Autodesk Inventor part; units mm, degrees
ref_plane "Work Plane1" through (-6.76, 0, 0) normal (-1, 0, 0) x (0, -1, 0)
ref_plane "XZ Plane" through (0, 0, 0) normal (0, 1, 0) x (-1, 0, 0)
ref_plane "XY Plane" through (0, 0, 0) normal (0, 0, 1) x (1, 0, 0)
sketch "Sketch1" plane through (0, 0, 0) normal (0, 0, 1) x (1, 0, 0)
  line L0 (0, 0) -> (0, 66.5)
  line L1 (3.2, 0) -> (4, 0)
  line L2 (4, 0) -> (4, 5.9)
  line L3 (4, 5.9) -> (3.4, 6.5)
  line L4 (3.4, 6.5) -> (3.4, 45.3)
  line L5 (3.4, 45.3) -> (4, 45.9)
  line L6 (4, 45.9) -> (4, 66.5)
  line L7 (4, 66.5) -> (3.2, 66.5)
  line L8 (3.2, 66.5) -> (3.2, 0)
  dimension "d0" = 45
  dimension "d1" = 45
  dimension "d2" = 6.4
  dimension "d3" = 8
  dimension "d4" = 6.5
  dimension "d5" = 45.3
  dimension "d6" = 66.5
  dimension "d7" = 6.8
revolve "Revolution1" add sketch "Sketch1" angle 360 about axis through (0, 0, 0) along (0, 1, 0)
ref_plane "Work Plane1" through (-6.76, 0, 0) normal (-1, 0, 0) x (0, -1, 0)
sketch "Sketch2" plane through (-6.76, 0, 0) normal (-1, 0, 0) x (0, -1, 0)
  line L0 (-65.7, 1.5) -> (-54.5, 1.5)
  line L1 (-54.5, 1.5) -> (-54.5, -1.5)
  line L2 (-54.5, -1.5) -> (-65.7, -1.5)
  line L3 (-65.7, -1.5) -> (-65.7, 1.5)
  line L4 (-65.7, 2.75) -> (-54.5, 2.75)
  line L5 (-54.5, 2.75) -> (-54.5, -2.75)
  line L6 (-54.5, -2.75) -> (-65.7, -2.75)
  line L7 (-65.7, -2.75) -> (-65.7, 2.75)
  line L8 (13.7787, 0) -> (-82.6723, 0)
  line L9 (0, -4) -> (0, 4)
  dimension "d10" = 54.5
  dimension "d11" = 65.7
  dimension "d12" = 5.5
  dimension "d13" = 3
extrude "Extrusion1" add sketch "Sketch2" against normal up to surface
extrude "Extrusion2" cut sketch "Sketch2" against normal blind 1 contours L7 L4 L5 L0 | L2 L5 L6 L7
sketch "Sketch3" plane through (-5.76, 0, 0) normal (-1, 0, 0) x (0, 0, 1)
  line L0 (-1.5, 65.7) -> (-1.5, 54.5)
  line L1 (-2.75, 65.7) -> (-1.5, 65.7)
  line L2 (-2.75, 54.5) -> (-2.75, 65.7)
  line L3 (-1.5, 54.5) -> (-2.75, 54.5)
  line L4 (1.5, 54.5) -> (1.5, 65.7)
  line L5 (2.75, 54.5) -> (1.5, 54.5)
  line L6 (2.75, 65.7) -> (2.75, 54.5)
  line L7 (1.5, 65.7) -> (2.75, 65.7)
  line L8 (-4, 66.5) -> (4, 66.5)
  line L9 (2.75, 65.7) -> (-2.75, 65.7)
  line L10 (-2.75, 65.7) -> (-2.75, 66.5)
  line L11 (-2.75, 66.5) -> (2.75, 66.5)
  line L12 (2.75, 66.5) -> (2.75, 65.7)
extrude "Extrusion3" add sketch "Sketch3" against normal up to surface contours L1 L10 L8 L12 L7 L9
sketch "Sketch4" plane through (0, 66.5, 0) normal (0, 1, 0) x (1, 0, 0)
  line L0 (-5.76, 1.5) -> (-5.76, 2.75)
  line L1 (-5.76, 2.25) -> (-4.06, 2.25)
  line L2 (-4.06, 2.25) -> (-4.06, -2.25)
  line L3 (-4.06, -2.25) -> (-5.76, -2.25)
  line L4 (-5.76, -2.75) -> (-5.76, 2.75)
  line L5 (-4.76, 2.25) -> (-4.76, -2.25)
  line L6 (-8.912, 0) -> (6.152, 0)
  line L7 (-5.76, 2.25) -> (-5.76, -2.25)
  point P0 (0, 0)
  dimension "d20" = 4.06
  dimension "d21" = 4.76
  dimension "d22" = 4.5
extrude "Extrusion4" cut sketch "Sketch4" against normal up to surface (0.8 mm away) contours L0 L1 L5 L6 L4 | L6 L5 L3 L4
extrude "Extrusion5" cut sketch "Sketch4" against normal blind 9 contours L1 L2 L6 L5 | L6 L2 L3 L5
equation "\"d1\" = d0"
properties part number "PP-12" material "ABS Plastic"
Model file for the job. Use its own axes, mm. A direction names the side the tool comes from. Give positions to 0.01 mm unless a question says otherwise; leave off trailing zeros. Loops run counter-clockwise (first coordinate to the right, second up) from the corner with the lowest first, then second, coordinate; pieces in that order, holes last.
1) Flat gauge pins, fed straight in: pin 1 Ø1 at (x, z) = (-6, 0.5) entering from +Y; pin 2 Ø2 at (x, y) = (-3.5, 7.5) entering from +Z; pin 3 Ø2 at (x, y) = (-2.5, 27) entering from +Z. Where does each tip first touch, or does it go through?
2) Saw through at D-D (y = 52.5). Write the cut outline in (x, z).
3) Saw through at C-C (y = 22). Write the cut outline in (x, z).
4) Saw through at B-B (z = 0). Write the cut outline in (x, y).
5) Pull direction Z, two halves, no side cores. Call faces 4 (the flat face through (-4, 61, 2.75)), 5 (the flat face through (-5.76, 61, -2)), 6 (the flat face through (-4.5, 62.1, 2.25)): +Z half, -Z half, draft (parallel to the pull), parting line (faces both ways), or undercut.
6) Tool access for faces 1 (the flat face through (-4.5, 62.1, -2.25)), 2 (the cylindrical face through (-0.74, 26.17, 3.32)), 3 (the cylindrical face through (3.695, 56.344, 1.532)): list every direction of +Z, -Z, +X, -X, +Y, -Y with a clear straight run to the whole face (end or side of a thin tool).
7) Wall check: line 1 (Z direction, x = 0, y = 39); line 2 (Z direction, x = 0, y = 52). Give the ranges that are in metal, low to high.
8) Saw through at A-A (x = 0). Write the cut outline in (y, z).
Answer block:
1. pin 1: stops at y = 65.7
1. pin 2: stops at z = 2.3
1. pin 3: stops at z = 3.05
2. outline: circle Ø8 at (0, 0); hole circle Ø6.4 at (0, 0)
3. outline: circle Ø6.8 at (0, 0); hole circle Ø6.4 at (0, 0)
4. outline: (-6.76, 54.5) - (-4, 54.5) - (-4, 45.9) - (-3.4, 45.3) - (-3.4, 6.5) - (-4, 5.9) - (-4, 0) - (-3.2, 0) - (-3.2, 66.5) - (-4.06, 66.5) - (-4.06, 57.5) - (-4.76, 57.5) - (-4.76, 65.7) - (-6.76, 65.7) - close; (3.2, 0) - (4, 0) - (4, 5.9) - (3.4, 6.5) - (3.4, 45.3) - (4, 45.9) - (4, 66.5) - (3.2, 66.5) - close
5. face 4: +Z half
5. face 5: draft
5. face 6: undercut
6. face 1: +Y
6. face 2: none
6. face 3: -Y
7. line 1: z = -3.4 to -3.2, 3.2 to 3.4
7. line 2: z = -4 to -3.2, 3.2 to 4
8. outline: (0, -4) - (5.9, -4) - (6.5, -3.4) - (45.3, -3.4) - (45.9, -4) - (66.5, -4) - (66.5, -3.2) - (0, -3.2) - close; (0, 3.2) - (66.5, 3.2) - (66.5, 4) - (45.9, 4) - (45.3, 3.4) - (6.5, 3.4) - (5.9, 4) - (0, 4) - close
